Answer from the drawing. Dimensions are ordinates in mm from the lowest x, y and z of the part. Give positions to 0.01 mm unless a question says otherwise; leave off trailing zeros. Loops run counter-clockwise (first coordinate to the right, second up) from the corner with the lowest first, then second, coordinate; pieces in that order, holes last. Notation, with made-up numbers: (-31, -24) -> (-14, -24) arc R26 ccw to (-14, 11) -> close; hole circle Ø5 at (32.5, 32.5). An arc over 180 degrees is marked (long way). Return JSON: item names as keys, results as strings. Group by question number.
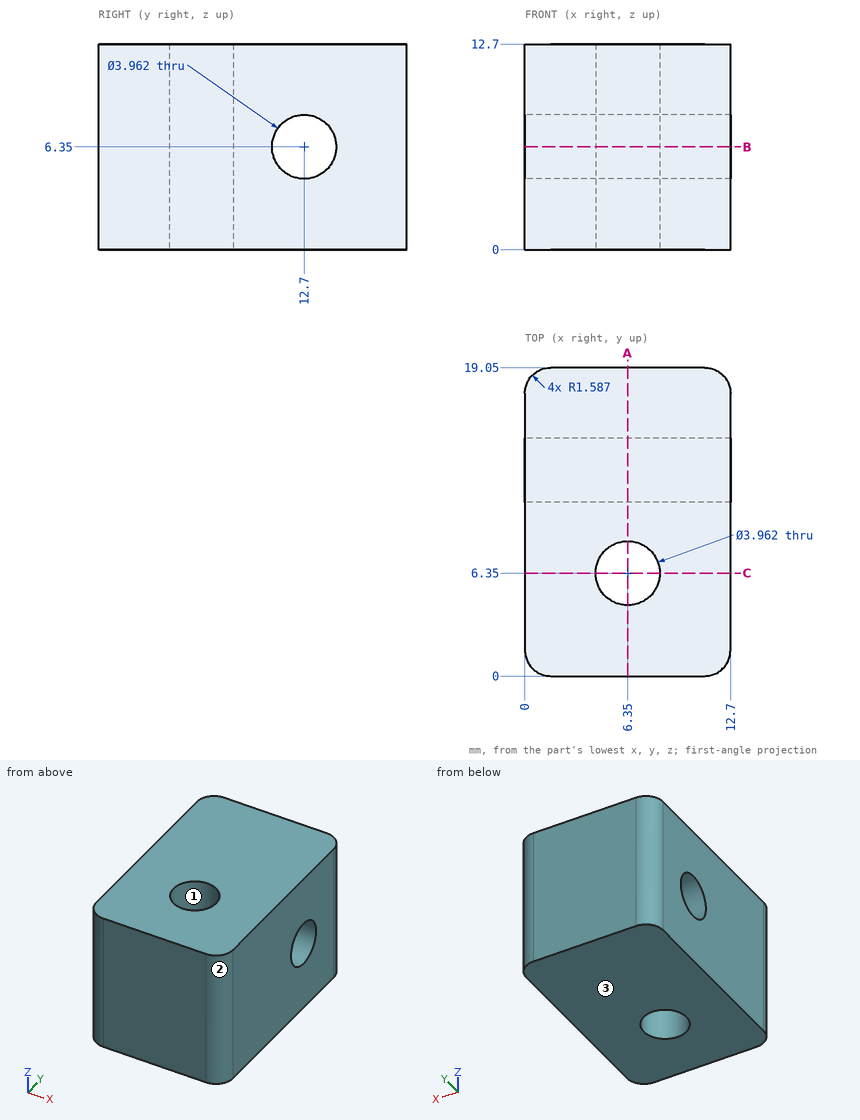
1. Section A-A on x = 6.35 is taken. Determine the outline of the cut face in (y, z).
2. Section C-C on y = 6.35 is taken. Determine the outline of the cut face in (x, z), then the cut area to 3 significant figures.
3. Straight lines are drawn through the part: line 1 (Z direction, x = 7.25, y = 12.7); line 2 (Z direction, x = 1, y = 11.75); line 3 (X direction, y = 1.5, z = 11.25). For each, find the intervals that lie inside material, in ascending order. Write a range as from..to.
4. Determine the mould class of the marked faces 1, 2 and 3 for opening direction X: pulls with the +X half, pulls with the -X half, needs draft (parallel to the pull), parting line crosses it, or undercut.
5. Section B-B on z = 6.35 is taken. State how many separate pieces and enclosed holes the cut face has, then the cut area to 3 significant figures.
Completed:
{
 "1": {"outline": "(0, 0) -> (4.37, 0) -> (4.37, 12.7) -> (0, 12.7) -> close; (8.33, 0) -> (19.05, 0) -> (19.05, 12.7) -> (8.33, 12.7) -> close; hole circle Ø3.96 at (12.7, 6.35)"},
 "2": {"outline": "(0, 0) -> (4.37, 0) -> (4.37, 12.7) -> (0, 12.7) -> close; (8.33, 0) -> (12.7, 0) -> (12.7, 12.7) -> (8.33, 12.7) -> close", "area": "111 mm²"},
 "3": {"line 1": "z = 0..4.37, 8.33..12.7", "line 2": "z = 0..4.61, 8.09..12.7", "line 3": "x = 0..12.7"},
 "4": {"face 1": "undercut", "face 2": "pulls with the +X half", "face 3": "needs draft"},
 "5": {"separate pieces": "2", "enclosed holes": "1", "area": "177 mm²"}
}
